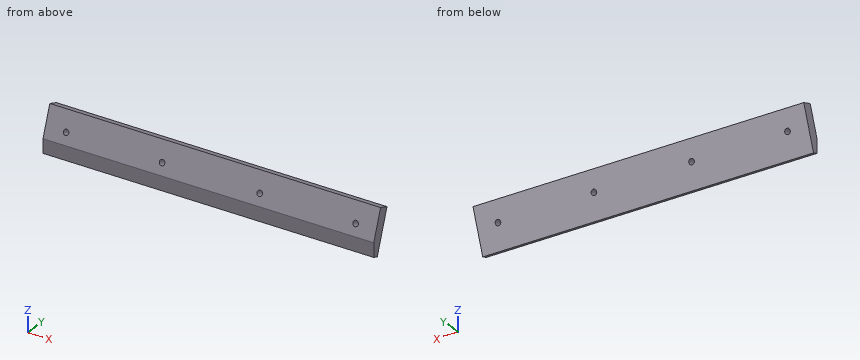
Solid Edge part; units mm, degrees
sketch "Sketch1" plane through (0, 0, 0) normal (1, 0, 0) x (0, 1, 0)
  line L0 (-53.0208, 191.8367) -> (-58.0424, 177.7797)
  line L1 (-58.0424, 177.7797) -> (-58.0424, 170.9866)
  line L2 (-58.0424, 170.9866) -> (-55.4859, 170.0733)
  line L3 (-48.3122, 190.1546) -> (-55.4859, 170.0733)
  line L4 (-53.0208, 191.8367) -> (-48.3122, 190.1546)
extrude "Protrusion1" add sketch "Sketch1" along normal mid plane 162
sketch "Sketch2" plane through (0, -51.8991, 180.114) normal (0, 0.9417, -0.3364) x (-1, 0, 0)
  circle A0 centre (-70.9, 1.1621) radius 1.35
  circle A1 centre (-23.9, 1.1621) radius 1.35
  circle A2 centre (23.9, 1.1621) radius 1.35
  circle A3 centre (70.9, 1.1621) radius 1.35
extrude "Cutout1" cut sketch "Sketch2" against normal up to next
Design review of the part built by this model. Coordinates are the model's own, in mm. Round coordinates to 2 decimals unless told otherwise and drop trailing zeros. Write each loop counter-clockwise with the first axis right and the second up, starting at its lowest first coordinate (ties: lowest second). Pieces come first, ordered by that corner, then holes.
Item 1: Wall thickness on L1, parallel to X at y = -56, z = 181.5; L2, parallel to X at y = -53.5, z = 183; L3, parallel to Y at x = -50.5, z = 177.25: over which ranges is each line inside the solid? List them lowest first.
Item 2: Consider section B-B on z = 174. Give the boundary of the cut face in (x, y).
Item 3: For pin 1 Ø3 at (x, z) = (57.5, 184) entering from -Y; pin 2 Ø1.5 at (x, y) = (44, -52) entering from +Z; pin 3 Ø1 at (x, z) = (26.5, 177.5) entering from +Y, all flat-tipped, find the tip position at first contact; note any pin that passes through.
Item 4: Consider section A-A on x = 51.5. Give the boundary of the cut face in (y, z), and give its area (3 significant figures).
Item 5: Consider section C-C on z = 188.25. Give the boundary of the cut face in (x, y).
Check values:
1. L1: x = -81 to -71.44, -70.36 to -24.44, -23.36 to 23.36, 24.44 to 70.36, 71.44 to 81
1. L2: x = -81 to -71.79, -70.01 to -24.79, -23.01 to 23.01, 24.79 to 70.01, 71.79 to 81
1. L3: y = -58.04 to -52.92
2. outline: (-81, -58.04) - (81, -58.04) - (81, -54.08) - (-81, -54.08) - close
3. pin 1: stops at y = -56.36
3. pin 2: stops at z = 191.74
3. pin 3: stops at y = -52.65
4. outline: (-58.04, 170.99) - (-55.49, 170.07) - (-48.31, 190.15) - (-53.02, 191.84) - (-58.04, 177.78) - close
4. area: 99.3 mm2
5. outline: (-81, -54.3) - (81, -54.3) - (81, -48.99) - (-81, -48.99) - close
